```python
from build123d import *

# Parameters (mm, degrees)
F1_DEPTH = 5.3
F2_R     = 4
F3_DEPTH = 60
F4_SIZE  = 1


with BuildPart() as f1:
    # F0 (on Front) → F1 (new body)
    with BuildSketch(Plane.XZ):
        Polygon((3.752777, -6.5), (7.505553, 0), (3.752777, 6.5), (-3.752777, 6.5), (-7.505553, 0), (-3.752777, -6.5), align=None)
    extrude(amount=F1_DEPTH)

    # F2 (on face) → F3 (join)
    with BuildSketch(Plane(origin=(0, 0, 0), x_dir=(-1, 0, 0), z_dir=(0, 1, 0))):
        Circle(F2_R)
    extrude(amount=F3_DEPTH)

    # F4
    f4_edges = [f1.edges().sort_by_distance(p)[0] for p in [
        (4, 60, 0),
    ]]
    chamfer(f4_edges, length=F4_SIZE)


solid = f1.part
```
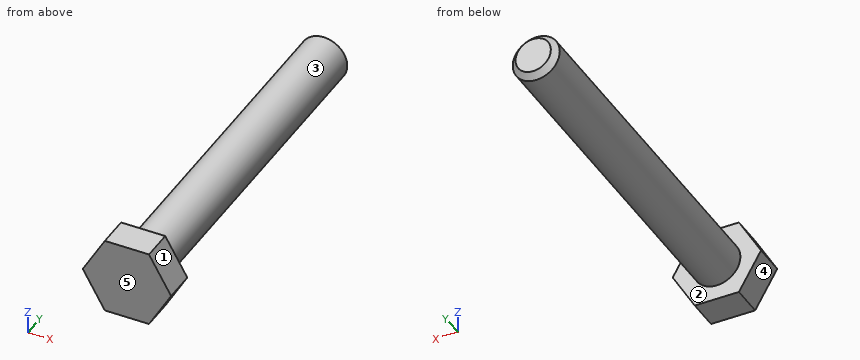
The listing builds one solid part. Answer for the finished solid, in the listing's coordinates (mm). Face numbers are marked on the shaded views. A direction names the side the tool comes from. Coordinates: 2 decimals unless noted, no trailing zeros. Write each loop counter-clockwise with the first axis right and the second up, starting at its lowest first coordinate (ties: lowest second). Pieces come first, ordered by that corner, then holes. Notation, with made-up numbers: (49, 62) - (68, 62) arc R14 ccw to (68, 76) - close; hole circle Ø11 at (36.5, 54.25). An arc over 180 degrees is marked (long way). Return JSON: item names as keys, results as strings. Group by question number.
1. A cutting plane is placed at B-B, the plane y = 22.5. Determine the outline of the cut face in (x, z), plus the area to 3 significant figures.
2. Straight lines are drawn through the part: L1, parallel to Y at x = 0, z = -4.75; L2, parallel to X at y = 6, z = -0.25; L3, parallel to X at y = 20.5, z = 2. For each, find the intervals that lie inside material, in ascending order.
3. A cutting plane is placed at A-A, the plane x = 0. Determine the outline of the cut face in (y, z), plus the area to 3 significant figures.
4. Given pin 1 (1.5 mm diameter, centred on y = 37.5, z = 4, fed in from +X); pin 2 (4 mm diameter, centred on y = 21, z = 1, fed in from +X); pin 3 (5 mm diameter, centred on y = 27, z = 2.5, fed in from -X), each flat-ended and moving along its own axis, determine where each tip first touches the part or whether it passes through.
5. Which of the six approach directions +Z, -Z, +X, -X, +Y, -Y give full straight-line access (tool end or side, diameter ignored) to the marked faces 1 and 2?
6. A cutting plane is placed at C-C, the plane z = 5.5. Determine the outline of the cut face in (x, y).
7. Determine the mould class of the marked faces 3, 4 and 5 for opening direction Z: released by +Z, released by -Z, zero draft, split by the parting line, or undercut.
Ans:
{
 "1": {"outline": "circle Ø8 at (0, 0)", "area": "50.3 mm²"},
 "2": {"L1": "-5.3 to 0", "L2": "-3.99 to 3.99", "L3": "-3.46 to 3.46"},
 "3": {"outline": "(-5.3, -6.5) - (0, -6.5) - (0, -4) - (59, -4) - (60, -3) - (60, 3) - (59, 4) - (0, 4) - (0, 6.5) - (-5.3, 6.5) - close", "area": "548 mm²"},
 "4": {"pin 1": "x = 2.33", "pin 2": "x = 4", "pin 3": "x = -4"},
 "5": {"face 1": "+Z, +X, +Y, -Y", "face 2": "+Y"},
 "6": {"outline": "(-4.33, -5.3) - (4.33, -5.3) - (4.33, 0) - (-4.33, 0) - close"},
 "7": {"face 3": "split by the parting line", "face 4": "released by -Z", "face 5": "zero draft"}
}
